from build123d import *

# Parameters (mm, degrees)
SKETCH1_W               = 21.333333334
SKETCH1_H               = 32
BOSS_EXTRUDE1_DEPTH     = 5
SKETCH2_W               = 37.6
SKETCH2_H               = 32
BOSS_EXTRUDE2_DEPTH     = 5
SKETCH7_R               = 1.3
CUT_EXTRUDE2_DEPTH      = 10
CUT_EXTRUDE3_DEPTH      = 51.465433715
CUT_EXTRUDE3_DEPTH_BACK = 51.465433715
SKETCH8_W               = 25.4
SKETCH8_H               = 1
SKETCH8_W_2             = 9
SKETCH8_H_2             = 2
SKETCH9_W               = 32.866666667
SKETCH9_H               = 32
BOSS_EXTRUDE3_DEPTH     = 3
CUT_EXTRUDE4_DEPTH      = 51.465433715
CUT_EXTRUDE4_DEPTH_BACK = 51.465433715
SKETCH10_R              = 3
CUT_EXTRUDE5_DEPTH      = 8
FILLET8_R               = 3
FILLET9_R               = 10
FILLET10_R              = 5


with BuildPart() as part:
    # Sketch1 → Boss-Extrude1 (new body)
    with BuildSketch(Plane(origin=(0, 0, 0), x_dir=(1, 0, 0), z_dir=(0, 1, 0))):
        Rectangle(SKETCH1_W, SKETCH1_H)
    extrude(amount=BOSS_EXTRUDE1_DEPTH)

    # Sketch2 → Boss-Extrude2 (add)
    with BuildSketch(Plane(origin=(0, 0, 0), x_dir=(1, 0, 0), z_dir=(0, 1, 0))):
        with Locations((28.8, 0)):
            Rectangle(SKETCH2_W, SKETCH2_H)
    extrude(amount=BOSS_EXTRUDE2_DEPTH)

    # Sketch7 → Cut-Extrude2 (cut)
    with BuildSketch(Plane(origin=(0, 0, 0), x_dir=(1, 0, 0), z_dir=(0, 1, 0))):
        with Locations(Location((38.4, -9.5, 0), (0, 0, 90))):
            Circle(SKETCH7_R)
        with Locations(Location((31.4, -5.5, 0), (0, 0, 90))):
            Circle(SKETCH7_R)
        with Locations(Location((38.4, 5.5, 0), (0, 0, 90))):
            Circle(SKETCH7_R)
        with Locations(Location((31.4, 9.5, 0), (0, 0, 90))):
            Circle(SKETCH7_R)
    extrude(amount=CUT_EXTRUDE2_DEPTH, mode=Mode.SUBTRACT)

    # Sketch8 → Cut-Extrude3 (cut, two sides: drawn at the far end of the back side and taken through both)
    with BuildSketch(Plane.XY.offset(-CUT_EXTRUDE3_DEPTH_BACK)):
        with Locations((34.9, 0.5)):
            Rectangle(SKETCH8_W, SKETCH8_H)
        with Locations((18.833333333, 4)):
            Rectangle(SKETCH8_W_2, SKETCH8_H_2)
    extrude(amount=CUT_EXTRUDE3_DEPTH + CUT_EXTRUDE3_DEPTH_BACK, mode=Mode.SUBTRACT)

    # Sketch9 → Boss-Extrude3 (add)
    with BuildSketch(Plane(origin=(0, 0, 0), x_dir=(1, 0, 0), z_dir=(0, 1, 0))):
        with Locations((5.766666667, 0)):
            Rectangle(SKETCH9_W, SKETCH9_H)
    extrude(amount=-BOSS_EXTRUDE3_DEPTH)

    # Sketch10 → Cut-Extrude4 (cut, two sides: drawn at the far end of the back side and taken through both)
    with BuildSketch(Plane(origin=(0, 0, 0), x_dir=(1, 0, 0), z_dir=(0, 1, 0)).offset(-CUT_EXTRUDE4_DEPTH_BACK)):
        with Locations(Location((-0.666666667, 8, 0), (0, 0, 270))):
            Circle(SKETCH10_R)
        with Locations(Location((-0.666666667, -8, 0), (0, 0, 270))):
            Circle(SKETCH10_R)
    extrude(amount=CUT_EXTRUDE4_DEPTH + CUT_EXTRUDE4_DEPTH_BACK, mode=Mode.SUBTRACT)

    # Sketch11 → Cut-Extrude5 (cut)
    with BuildSketch(Plane(origin=(0, 0, 0), x_dir=(1, 0, 0), z_dir=(0, 1, 0))):
        with BuildLine():
            Line((-5.866666667, 8), (-5.866666667, -8))
            ThreePointArc((-5.866666667, -8), (-0.666666667, -13.2), (4.533333333, -8))
            Line((4.533333333, -8), (4.533333333, 8))
            ThreePointArc((4.533333333, 8), (-0.666666667, 13.2), (-5.866666667, 8))
        make_face()
    extrude(amount=-CUT_EXTRUDE5_DEPTH, mode=Mode.SUBTRACT)

    # Fillet8
    # the kernel refuses this fillet: 3 mm, written as the material it takes off along each edge
    with BuildSketch(Plane(origin=(-0.666666667, -3, -8), x_dir=(1, 0, 0), z_dir=(0, 0, 1))) as fillet8_piece_1:
        with BuildLine():
            CenterArc((5.2 + FILLET8_R, FILLET8_R), FILLET8_R, 180, 90)
            Line((5.2, FILLET8_R), (5.2, 0))
            Line((5.2, 0), (5.2 + FILLET8_R, 0))
        make_face()
    revolve(axis=Axis((-0.666666667, -3, -8), (0, 1, 0)), revolution_arc=180, mode=Mode.SUBTRACT)
    with BuildSketch(Plane(origin=(-0.666666667, -3, 8), x_dir=(-1, 0, 0), z_dir=(0, 0, -1))) as fillet8_piece_2:
        with BuildLine():
            CenterArc((5.2 + FILLET8_R, FILLET8_R), FILLET8_R, 180, 90)
            Line((5.2, FILLET8_R), (5.2, 0))
            Line((5.2, 0), (5.2 + FILLET8_R, 0))
        make_face()
    revolve(axis=Axis((-0.666666667, -3, 8), (0, 1, 0)), revolution_arc=180, mode=Mode.SUBTRACT)
    with BuildSketch(Plane(origin=(-5.866666667, -3, 8), x_dir=(-1, 0, 0), z_dir=(0, 0, -1)), Plane(origin=(4.533333333, -3, -8), x_dir=(1, 0, 0), z_dir=(0, 0, 1))) as fillet8_piece_3:
        with BuildLine():
            CenterArc((FILLET8_R, FILLET8_R), FILLET8_R, 180, 90)
            Line((0, FILLET8_R), (0, 0))
            Line((0, 0), (FILLET8_R, 0))
        make_face()
    extrude(amount=16, mode=Mode.SUBTRACT)

    # Fillet9
    # the kernel refuses this fillet: 10 mm, written as the material it takes off along each edge
    with BuildSketch(Plane(origin=(23.333333333, 5, 31), x_dir=(0, -1, 0), z_dir=(0, 0, -1))) as fillet9_piece_1:
        with BuildLine():
            CenterArc((10, -6), FILLET9_R, 143.130102354, 36.869897646)
            Line((0, -6), (-0.2, -6))
            Line((-0.2, -6), (-0.2, 0))
            Line((-0.2, 0), (0, 0.2))
            ThreePointArc((0, 0.2), (1, 0.2), (1.84, 0.12))
            Line((1.84, 0.12), (2, 0))
        make_face()
    extrude(amount=62, mode=Mode.SUBTRACT)
    with BuildSketch(Plane(origin=(14.333333333, 5, -31), x_dir=(-1, 0, 0), z_dir=(0, 0, 1))) as fillet9_piece_2:
        with BuildLine():
            CenterArc((6, 10), FILLET9_R, 233.130102354, 36.869897646)
            Line((0, 2), (-0.12, 1.84))
            ThreePointArc((-0.12, 1.84), (-0.2, 1), (-0.2, 0))
            Line((-0.2, 0), (0, -0.2))
            Line((0, -0.2), (6, -0.2))
            Line((6, -0.2), (6, 0))
        make_face()
    extrude(amount=62, mode=Mode.SUBTRACT)
    with BuildSketch(Plane(origin=(22.2, -3, -36), x_dir=(0, 1, 0), z_dir=(0, 0, 1))) as fillet9_piece_3:
        with BuildLine():
            CenterArc((10, 8), FILLET9_R, 180, 53.130102354)
            Line((0, 8), (-0.2, 8))
            Line((-0.2, 8), (-0.2, 0))
            Line((-0.2, 0), (0, -0.2))
            ThreePointArc((0, -0.2), (2, -0.2), (3.88, -0.16))
            Line((3.88, -0.16), (4, 0))
        make_face()
    extrude(amount=72, mode=Mode.SUBTRACT)

    # Fillet10
    fillet10_edges = [part.edges().sort_by_distance(p)[0] for p in [
        (22.2, 1, 0),
        (14.333333333, 3, 0),
        (23.333333333, 3, 0),
    ]]
    fillet(fillet10_edges, radius=FILLET10_R)


solid = part.part
Geometry check sheet. Reference: the model listing, model coordinates, mm. A direction names the side the tool comes from. Give positions to 0.01 mm unless a question says otherwise; leave off trailing zeros. Order: outer loops, then holes, each group sorted by start corner. A loop starts at its lowest first (then second) coordinate and runs counter-clockwise, first axis right, second up.
1. Scan lines: line 1 (Z direction, x = 31.5, y = 3.5); line 2 (X direction, y = 3.75, z = 8); line 3 (X direction, y = 1.9, z = 5.5). Record each from-to range of solid material in increasing order.
Completed:
line 1: z = -16 to -10.8, -8.2 to 4.2, 6.8 to 16
line 2: x = -10.67 to -3.67, 2.33 to 13.17, 24.49 to 47.6
line 3: x = -10.67 to -2.32, 0.99 to 30.1, 32.7 to 47.6
2. Sectioned sample at B-B (x = 38.4). Record the boundary of the cut face in (y, z).
Completed:
outline: (1, -16) - (5, -16) - (5, -6.8) - (1, -6.8) - close; (1, -4.2) - (5, -4.2) - (5, 8.2) - (1, 8.2) - close; (1, 10.8) - (5, 10.8) - (5, 16) - (1, 16) - close
3. Sectioned sample at D-D (y = 2.25). Record the boundary of the cut face in (x, z).
Completed:
outline: (-10.67, -16) - (47.6, -16) - (47.6, 16) - (-10.67, 16) - close; hole circle Ø6 at (-0.67, -8); hole circle Ø6 at (-0.67, 8); hole circle Ø2.6 at (31.4, -9.5); hole circle Ø2.6 at (31.4, 5.5); hole circle Ø2.6 at (38.4, -5.5); hole circle Ø2.6 at (38.4, 9.5)
4. Sectioned sample at C-C (z = 6). Record the boundary of the cut face in (x, y).
Completed:
outline: (-10.67, -3) - (-8.87, -3) arc R3 ccw to (-5.87, 0) - (-2.9, 0) - (-2.9, 5) - (-10.67, 5) - close; (1.57, 0) - (4.53, 0) arc R3 ccw to (7.53, -3) - (14.2, -3) arc R10 ccw to (21, -0.33) arc R5 cw to (24.4, 1) - (30.2, 1) - (30.2, 5) - (29.33, 5) arc R10 ccw to (24.34, 3.67) arc R5 cw to (21.85, 3) - (15.82, 3) arc R5 cw to (13.32, 3.67) arc R10 ccw to (8.33, 5) - (1.57, 5) - close; (32.6, 1) - (47.6, 1) - (47.6, 5) - (32.6, 5) - close
5. Draft check along Z on faces 6 (the face through (-1, 5, 0)), 7 (the face through (12, 1, 16)), 8 (the face through (0.234, 2.465, -5.139)). Enter one of: pulls with the +Z half, pulls with the -Z half, needs draft (parallel to the pull), parting line crosses it, or undercut.
Completed:
face 6: needs draft
face 7: pulls with the +Z half
face 8: undercut
6. Depth check by flat-ended pin: pin 1 (5 mm diameter, centred on x = 1.5, z = 0.5, fed in from -Y); pin 2 (5 mm diameter, centred on x = 19, z = 0, fed in from +Y); pin 3 (12 mm diameter, centred on x = 24.5, z = 1, fed in from +Y). Enter the tip coordinate at first touch or a pass-through.
Completed:
pin 1: stops at y = 0
pin 2: stops at y = 3
pin 3: stops at y = 5
7. Access from +Z, -Z, +X, -X, +Y, -Y to the whole of each face (thin tool, end or side, straight path). Record for faces 1 (the face through (32.553, 2.972, 4.9)), 2 (the face through (5.39, -2.1, -0.11)), 3 (the face through (38, 5, 0)), 4 (the face through (36, 1, 0)), 5 (the face through (26.716, 4.651, 0.224)).
Completed:
face 1: +Y, -Y
face 2: -Y
face 3: +Z, -Z, +X, -X, +Y
face 4: +Z, -Z, +X, -Y
face 5: +Z, -Z, +Y
8. Sectioned sample at A-A (z = 2). Record the boundary of the cut face in (x, y).
Completed:
outline: (-10.67, -3) - (-8.87, -3) arc R3 ccw to (-5.87, 0) - (4.53, 0) arc R3 ccw to (7.53, -3) - (14.2, -3) arc R10 ccw to (21, -0.33) arc R5 cw to (24.4, 1) - (47.6, 1) - (47.6, 5) - (29.33, 5) arc R10 ccw to (24.34, 3.67) arc R5 cw to (21.85, 3) - (15.82, 3) arc R5 cw to (13.32, 3.67) arc R10 ccw to (8.33, 5) - (-10.67, 5) - close
